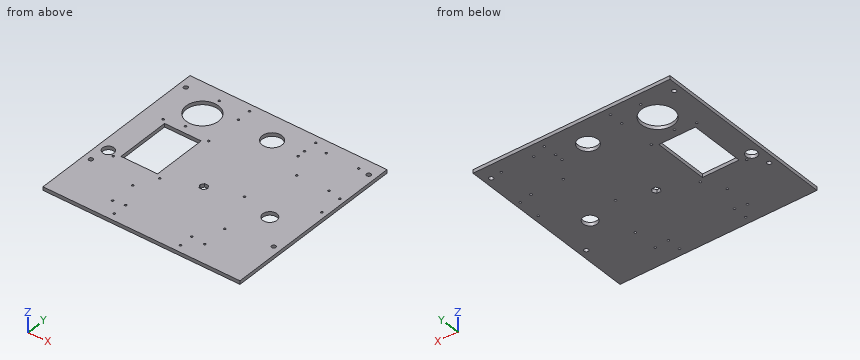
from build123d import *

# Parameters (mm, degrees)
ESQUISSE1_W              = 280
ESQUISSE1_H              = 210
BOSS_EXTRU_1_DEPTH       = 5
ESQUISSE2_R              = 3
ESQUISSE2_R_2            = 1.5
ESQUISSE2_R_3            = 8
ESQUISSE2_R_4            = 14
ESQUISSE2_R_5            = 10
ESQUISSE2_W              = 52
ESQUISSE2_H              = 78
ENL_V_MAT_EXTRU_1_DEPTH  = 351.035712464
ESQUISSE5_R              = 1.5
ENL_V_MAT_EXTRU_3_DEPTH  = 351.035712464
ESQUISSE6_W              = 280
ESQUISSE6_H              = 53
BOSS_EXTRU_4_DEPTH       = 5
ESQUISSE7_R              = 1.5
ENL_V_MAT_EXTRU_4_DEPTH  = 351.035712464
ESQUISSE8_R              = 1.5
ENL_V_MAT_EXTRU_5_DEPTH  = 351.035712464
ESQUISSE9_R              = 1.5
ENL_V_MAT_EXTRU_6_DEPTH  = 351.035712464
ESQUISSE14_R             = 23
ESQUISSE14_R_2           = 1.5
ENL_V_MAT_EXTRU_11_DEPTH = 351.035712464
ESQUISSE15_R             = 1.5
ENL_V_MAT_EXTRU_12_DEPTH = 351.035712464


with BuildPart() as part:
    # Esquisse1 → Boss.-Extru.1 (new body)
    with BuildSketch(Plane.XY):
        with Locations((140, 105)):
            Rectangle(ESQUISSE1_W, ESQUISSE1_H)
    extrude(amount=BOSS_EXTRU_1_DEPTH)

    # Esquisse2 → Enlèv. mat.-Extru.1 (cut, through all)
    with BuildSketch(Plane.XY):
        with Locations((270, 190)):
            Circle(ESQUISSE2_R)
        with Locations((10, 190)):
            Circle(ESQUISSE2_R)
        with Locations((10, 20)):
            Circle(ESQUISSE2_R)
        with Locations((270, 20)):
            Circle(ESQUISSE2_R)
        with Locations((187, 168)):
            Circle(ESQUISSE2_R_2)
        with Locations((187, 72)):
            Circle(ESQUISSE2_R_2)
        with Locations((91.5, 128)):
            Circle(ESQUISSE2_R_2)
        with Locations((27, 128)):
            Circle(ESQUISSE2_R_2)
        with Locations((92, 40)):
            Circle(ESQUISSE2_R_2)
        with Locations((26, 40)):
            Circle(ESQUISSE2_R_2)
        with Locations((15, 45)):
            Circle(ESQUISSE2_R_3)
        with Locations((146.093717203, 173)):
            Circle(ESQUISSE2_R_4)
        with Locations((232.477054828, 60.19739042)):
            Circle(ESQUISSE2_R_5)
        with Locations((272.5, 103)):
            Circle(ESQUISSE2_R_2)
        with Locations((272.5, 135)):
            Circle(ESQUISSE2_R_2)
        with Locations((59, 84)):
            Rectangle(ESQUISSE2_W, ESQUISSE2_H)
        Polygon((137.113248654, 63.5), (134.226497308, 58.5), (137.113248654, 53.5), (142.886751346, 53.5), (145.773502692, 58.5), (142.886751346, 63.5), align=None)
    extrude(amount=ENL_V_MAT_EXTRU_1_DEPTH, mode=Mode.SUBTRACT)

    # Esquisse5 → Enlèv. mat.-Extru.3 (cut, through all)
    with BuildSketch(Plane(origin=(0, 0, 0), x_dir=(-1, 0, 0), z_dir=(0, 0, -1))):
        with Locations((-93, 179.4)):
            Circle(ESQUISSE5_R)
        with Locations((-93, 199.4)):
            Circle(ESQUISSE5_R)
        with Locations((-187, 199.4)):
            Circle(ESQUISSE5_R)
        with Locations((-187, 179.4)):
            Circle(ESQUISSE5_R)
    extrude(amount=-ENL_V_MAT_EXTRU_3_DEPTH, mode=Mode.SUBTRACT)

    # Esquisse6 → Boss.-Extru.4 (add)
    with BuildSketch(Plane(origin=(0, 0, 0), x_dir=(-1, 0, 0), z_dir=(0, 0, -1))):
        with Locations((-140, -26.5)):
            Rectangle(ESQUISSE6_W, ESQUISSE6_H)
    extrude(amount=-BOSS_EXTRU_4_DEPTH)

    # Esquisse7 → Enlèv. mat.-Extru.4 (cut, through all)
    with BuildSketch(Plane(origin=(0, 0, 0), x_dir=(-1, 0, 0), z_dir=(0, 0, -1))):
        with Locations((-76.485302695, 11.149215752)):
            Circle(ESQUISSE7_R)
        with Locations((-76.473346209, -24.834750392)):
            Circle(ESQUISSE7_R)
    extrude(amount=-ENL_V_MAT_EXTRU_4_DEPTH, mode=Mode.SUBTRACT)

    # Esquisse8 → Enlèv. mat.-Extru.5 (cut, through all)
    with BuildSketch(Plane(origin=(0, 0, 0), x_dir=(-1, 0, 0), z_dir=(0, 0, -1))):
        with Locations((-206.944892865, -24.14)):
            Circle(ESQUISSE8_R)
        with Locations((-206.944892865, 11.843968131)):
            Circle(ESQUISSE8_R)
    extrude(amount=-ENL_V_MAT_EXTRU_5_DEPTH, mode=Mode.SUBTRACT)

    # Esquisse9 → Enlèv. mat.-Extru.6 (cut, through all)
    with BuildSketch(Plane(origin=(0, 0, 0), x_dir=(-1, 0, 0), z_dir=(0, 0, -1))):
        with Locations((-93, -22.4)):
            Circle(ESQUISSE9_R)
        with Locations((-93, -42.4)):
            Circle(ESQUISSE9_R)
        with Locations((-187, -42.4)):
            Circle(ESQUISSE9_R)
        with Locations((-187, -22.4)):
            Circle(ESQUISSE9_R)
    extrude(amount=-ENL_V_MAT_EXTRU_6_DEPTH, mode=Mode.SUBTRACT)

    # Esquisse14 → Enlèv. mat.-Extru.11 (cut, through all)
    with BuildSketch(Plane(origin=(0, 0, 0), x_dir=(-1, 0, 0), z_dir=(0, 0, -1))):
        with Locations((-54.48265068, 163.570126578)):
            Circle(ESQUISSE14_R)
        with Locations((-54.649127802, 193.569664664)):
            Circle(ESQUISSE14_R_2)
        with Locations((-54.316173557, 133.570588492)):
            Circle(ESQUISSE14_R_2)
    extrude(amount=-ENL_V_MAT_EXTRU_11_DEPTH, mode=Mode.SUBTRACT)

    # Esquisse15 → Enlèv. mat.-Extru.12 (cut, through all)
    with BuildSketch(Plane.XY.offset(5)):
        with Locations((254, 192)):
            Circle(ESQUISSE15_R)
        with Locations((208, 192)):
            Circle(ESQUISSE15_R)
        with Locations((208, 139)):
            Circle(ESQUISSE15_R)
        with Locations((254, 139)):
            Circle(ESQUISSE15_R)
    extrude(amount=-ENL_V_MAT_EXTRU_12_DEPTH, mode=Mode.SUBTRACT)


solid = part.part
Could you check a few things on this model? Use its own coordinates, in mm. Round coordinates to 2 decimals unless told otherwise and drop trailing zeros. Write each loop counter-clockwise with the first axis right and the second up, starting at its lowest first coordinate (ties: lowest second). Pieces come first, ordered by that corner, then holes. Notation, with made-up numbers: (1, 53) -> (50, 53) arc R20 cw to (50, 77) -> close; hole circle Ø4 at (26, -7). An arc over 180 degrees is marked (long way). Use a Markdown table: item, result.
1. For pin 1 Ø5 at (x, y) = (44, 42) entering from -Z, with a flat end and sliding along its axis, tell me the tip position at first contact or that it passes through.
Answer key:
| item | result |
|---|---|
| pin 1 | stops at z = 0 |
2. If we section it at B-B (y = 144): List the corners of the cut face in (x, z) for me, then the cut area to 3 significant figures.
Answer key:
| item | result |
|---|---|
| outline | (0, 0) -> (42.4, 0) -> (42.4, 5) -> (0, 5) -> close; (66.57, 0) -> (280, 0) -> (280, 5) -> (66.57, 5) -> close |
| area | 1,280 mm^2 |
3. If we section it at A-A (x = 18): List the corners of the cut face in (y, z) for me.
Answer key:
| item | result |
|---|---|
| outline | (-53, 0) -> (37.58, 0) -> (37.58, 5) -> (-53, 5) -> close; (52.42, 0) -> (210, 0) -> (210, 5) -> (52.42, 5) -> close |
4. Please list where these lines run through material, in increasing order: probe 1 along X at (y, z) = (199.4, 2); probe 2 along X at (y, z) = (20, 2.75); probe 3 along Y at (x, z) = (45, 2.6).
Answer key:
| item | result |
|---|---|
| probe 1 | x = 0 to 91.5, 94.5 to 185.5, 188.5 to 280 |
| probe 2 | x = 0 to 7, 13 to 267, 273 to 280 |
| probe 3 | y = -53 to 45, 123 to 142.62, 184.52 to 210 |
5. If we section it at C-C (z = 0.8): State how many separate pieces and enclosed holes the cut face has, then the cut area to 3 significant figures.
Answer key:
| item | result |
|---|---|
| separate pieces | 1 |
| enclosed holes | 36 |
| area | 66,400 mm^2 |
